The figure shows three views and two pictorial views of one solid part (mm, origin at its lowest corner). Answer the questions. A direction names the side the tool comes from. Round coordinates to 2 decimals unless told otherwise and drop trailing zeros. Order: outer loops, then holes, each group sorted by start corner. A loop starts at its lowest first (then second) coordinate and runs counter-clockwise, first axis right, second up. Notation, with made-up numbers: M -37,-21.5 L 0,-21.5 A36 ccw 0,16.5 Z; hole C 35,-27.5 d9. An arc over 180 degrees is marked long. Return JSON: item names as keys, results as strings.
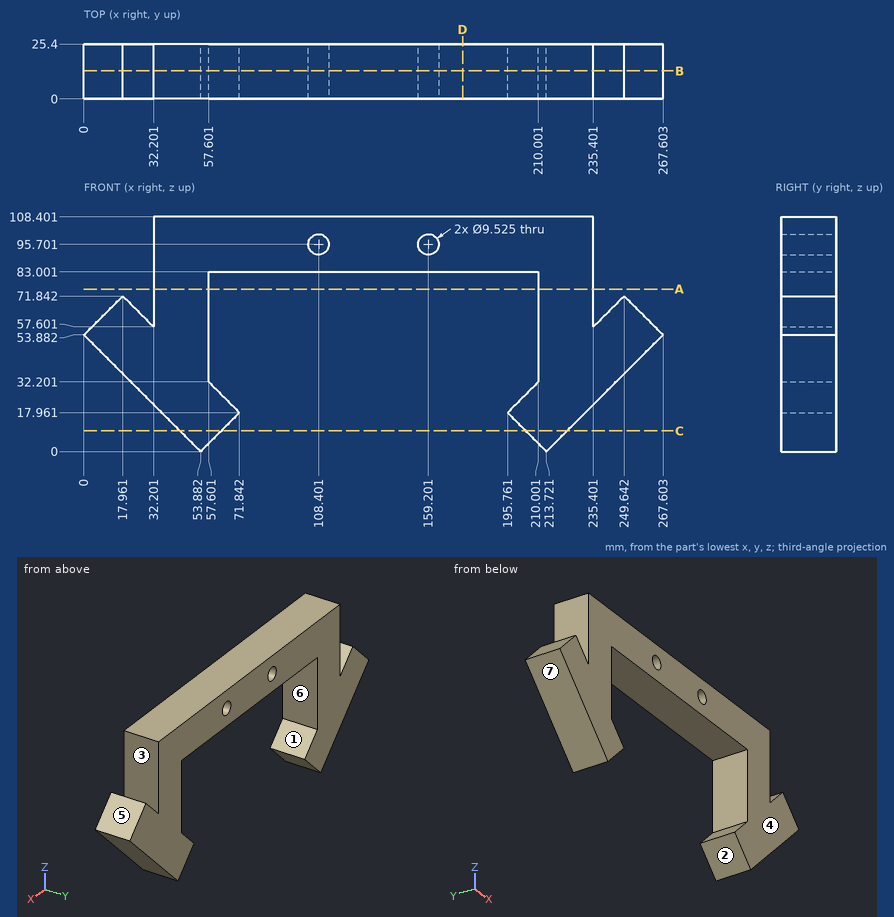
Item 1: Which of the six approach directions +Z, -Z, +X, -X, +Y, -Y give full straight-line access (tool end or side, diameter ignored) to the marked faces 1, 2, 3 and 4?
Output:
{"face 1": "+Y, -Y", "face 2": "-Z, +Y, -Y", "face 3": "+Z, +Y, -Y", "face 4": "+Z, -Z, +X, -X, -Y"}
Item 2: Find section C-C (z = 9.5). Determine the outline of the cut face in (x, y).
Output:
{"outline": "M 44.38,0 L 63.38,0 L 63.38,25.4 L 44.38,25.4 Z; M 204.22,0 L 223.22,0 L 223.22,25.4 L 204.22,25.4 Z"}
Item 3: Consider line 1 along X through (y, z) = (1.75, 86.5); line 2 along X through (y, z) = (2, 77); line 3 along Z through (x, y) = (122, 6). Determine where each line is inside the solid, lowest interval first. Write a range as [from, to].
Output:
{"line 1": "x = [32.2, 235.4]", "line 2": "x = [32.2, 57.6], [210, 235.4]", "line 3": "z = [83, 108.4]"}
Item 4: Find section A-A (z = 75). Determine the outline of the cut face in (x, y).
Output:
{"outline": "M 32.2,0 L 57.6,0 L 57.6,25.4 L 32.2,25.4 Z; M 210,0 L 235.4,0 L 235.4,25.4 L 210,25.4 Z"}
Item 5: Each of these flat-tipped pins is pushed along its axis until it touches: pin 1 (1 mm diameter, centred on y = 13, z = 78, fed in from -X); pin 2 (12 mm diameter, centred on y = 17.5, z = 25.5, fed in from +X); pin 3 (10 mm diameter, centred on y = 12, z = 22, fed in from -X); pin 4 (7.5 mm diameter, centred on x = 108.4, z = 95.7, fed in from -Y). Where does it stop, or does it pass through?
Output:
{"pin 1": "stops at x = 32.2", "pin 2": "stops at x = 245.22", "pin 3": "stops at x = 26.88", "pin 4": "passes through"}
Item 6: Find section B-B (y = 13). Determine the outline of the cut face in (x, z) (1 decimal), plus the area to 3 significant figures.
Output:
{"outline": "M 0,53.9 L 53.9,0 L 71.8,18 L 57.6,32.2 L 57.6,83 L 210,83 L 210,32.2 L 195.8,18 L 213.7,0 L 267.6,53.9 L 249.6,71.8 L 235.4,57.6 L 235.4,108.4 L 32.2,108.4 L 32.2,57.6 L 18,71.8 Z; hole C 108.4,95.7 d9.5; hole C 159.2,95.7 d9.5", "area": "10,800 mm^2"}
Item 7: The mould has two halves that part along X. Classify the marked faces 5, 6 and 7: pulls with the +X half, pulls with the -X half, needs draft (parallel to the pull), parting line crosses it, or undercut.
Output:
{"face 5": "pulls with the +X half", "face 6": "undercut", "face 7": "pulls with the -X half"}
Item 8: Find section D-D (x = 175). Determine the outline of the cut face in (y, z).
Output:
{"outline": "M 0,83 L 25.4,83 L 25.4,108.4 L 0,108.4 Z"}
